Could you check a few things on this drawing? It's one solid part, dimensions in mm from its lowest x, y, z. A direction names the side the tool comes from. Round coordinates to 2 decimals unless told otherwise and drop trailing zeros. Write each loop counter-clockwise with the first axis right and the second up, starting at its lowest first coordinate (ties: lowest second). Pieces come first, ordered by that corner, then holes. Notation, with made-up numbers: (15.5, -33) - (25.5, -33) arc R30 ccw to (25.5, -1) - close; hole circle Ø2 at (-39, 11.25). An arc over 180 degrees is marked (long way). Use one line per item in the form item = value. Start each with the question number.
1. Which directions (+Z, -Z, +X, -X, +Y, -Y) give clear straight access to the entire face, cutting with the end or side of a thin tool? Please do the marked faces 1, 2 and 3.
2. We'd pull the mould along X, two halves only. Please class the marked faces 4 and 5: +X half, -X half, draft (parallel to the pull), parting line (faces both ways), or undercut.
3. I want a section at B-B, the plane y = 30. List the corners of the cut face in (x, z) for me.
4. Will these pins go through, and if not, where does the flat tip stop? pin 1 (3 mm diameter, centred on x = 41.5, z = 8, fed in from -Y) (1 decimal); pin 2 (3 mm diameter, centred on y = 40.5, z = 14, fed in from -X); pin 3 (3.5 mm diameter, centred on x = 30, y = 23.5, fed in from -Z).
5. I want a section at A-A, the plane z = 18.25. State how many separate pieces and enclosed holes the cut face has, plus the area to 4 significant figures.
6. I want a section at C-C, the plane y = 36.5. List the corners of the cut face in (x, z) for me, plus the area to 3 significant figures.
7. If I drill on line 1 along Y through (x, z) = (31, 19.25) (1 decimal); line 2 along Y through (x, z) = (30, 8.5); line 3 along X through (y, z) = (29, 19.75) (1 decimal), over which ranges is the centre line in solid material (lowest first)?
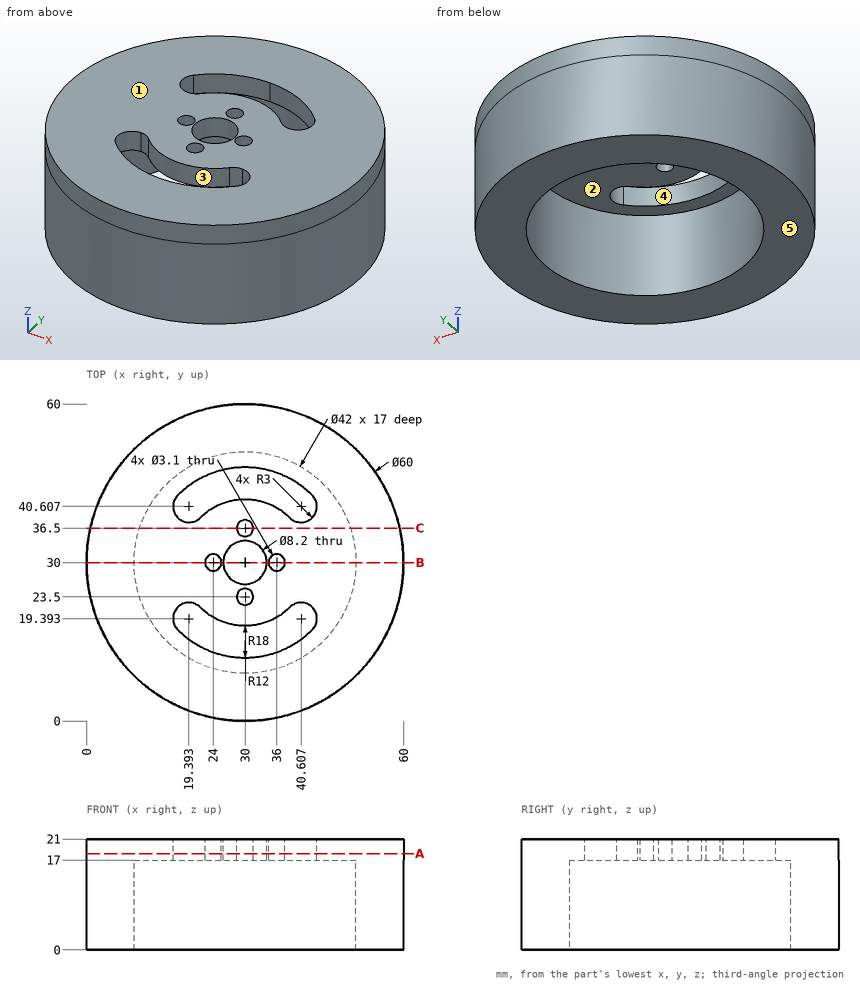
Model answer:
q1.face_1 = +Z, +X, -X, +Y, -Y
q1.face_2 = -Z
q1.face_3 = +Z, -Z
q2.face_4 = undercut
q2.face_5 = draft
q3.outline = (0, 0) - (9, 0) - (9, 17) - (22.45, 17) - (22.45, 21) - (0, 21) - close; (25.55, 17) - (25.9, 17) - (25.9, 21) - (25.55, 21) - close; (34.1, 17) - (34.45, 17) - (34.45, 21) - (34.1, 21) - close; (37.55, 17) - (51, 17) - (51, 0) - (60, 0) - (60, 21) - (37.55, 21) - close
q4.pin_1 = 1.7
q4.pin_2 = 1.38
q4.pin_3 = 17
q5.separate_pieces = 1
q5.enclosed_holes = 7
q5.area = 2,405 mm2
q6.outline = (0.71, 0) - (10.03, 0) - (10.03, 17) - (28.45, 17) - (28.45, 21) - (0.71, 21) - close; (31.55, 17) - (49.97, 17) - (49.97, 0) - (59.29, 0) - (59.29, 21) - (31.55, 21) - close
q6.area = 539 mm2
q7.line_1 = 0 to 12, 18 to 22.3, 24.7 to 26, 34 to 35.3, 37.7 to 42, 48 to 60
q7.line_2 = 0 to 9, 51 to 60
q7.line_3 = 0 to 22.8, 25.2 to 26, 34 to 34.8, 37.2 to 60
